The model under review builds one solid part; all positions refer to its coordinate system, in mm. A direction names the side the tool comes from. Round coordinates to 2 decimals unless told otherwise and drop trailing zeros. Order: outer loops, then holes, each group sorted by start corner. A loop starts at its lowest first (then second) coordinate and runs counter-clockwise, first axis right, second up.
from build123d import *

# Parameters (mm, degrees)
SKETCH_1_W      = 23
SKETCH_1_H      = 12.5
EXTRUDE_1_DEPTH = 20
SKETCH_2_W      = 32
SKETCH_2_H      = 12.5
SKETCH_2_R      = 1
EXTRUDE_2_DEPTH = 3
SKETCH_4_R      = 6.25
EXTRUDE_3_DEPTH = 6
SKETCH_5_R      = 2
EXTRUDE_4_DEPTH = 4


with BuildPart() as part:
    # 草图1 → 凸台-拉伸1 (new body)
    with BuildSketch(Plane(origin=(0, 0, 0), x_dir=(1, 0, 0), z_dir=(0, 1, 0))):
        Rectangle(SKETCH_1_W, SKETCH_1_H)
    extrude(amount=EXTRUDE_1_DEPTH)

    # 草图2 → 凸台-拉伸2 (add)
    with BuildSketch(Plane(origin=(0, 20, 0), x_dir=(1, 0, 0), z_dir=(0, 1, 0))):
        Rectangle(SKETCH_2_W, SKETCH_2_H)
        with Locations(Location((13.85, 0, 0), (0, 0, 270))):
            Circle(SKETCH_2_R, mode=Mode.SUBTRACT)
        with Locations(Location((-13.85, 0, 0), (0, 0, 90))):
            Circle(SKETCH_2_R, mode=Mode.SUBTRACT)
    extrude(amount=EXTRUDE_2_DEPTH)

    # 草图4 → 凸台-拉伸3 (add)
    with BuildSketch(Plane(origin=(0, 23, 0), x_dir=(1, 0, 0), z_dir=(0, 1, 0))):
        with Locations(Location((5.25, 0, 0), (0, 0, 270))):
            Circle(SKETCH_4_R)
    extrude(amount=EXTRUDE_3_DEPTH)

    # 草图5 → 凸台-拉伸4 (add)
    with BuildSketch(Plane(origin=(0, 29, 0), x_dir=(1, 0, 0), z_dir=(0, 1, 0))):
        with Locations(Location((5.25, 0, 0), (0, 0, 270))):
            Circle(SKETCH_5_R)
    extrude(amount=EXTRUDE_4_DEPTH)


solid = part.part
(1) We need section B-B (z = 0). Give the boundary of the cut face in (x, y), and give its area (3 significant figures).
(2) Tool access review of faces 5 (the flat face through (3, 29, 0)), 6 (the flat face through (-11.5, 10, 0)), 7 (the flat face through (12.7, 20, -0.1)), 8 (the flat face through (-16, 21, 0)): name each direction out of +Z, -Z, +X, -X, +Y, -Y from which nothing blocks a thin tool from reaching the whole face with its end or side.
(3) We need section C-C (x = 1.5). Give the boundary of the cut face in (y, z), and give its area (4 significant figures).
(4) We need section D-D (y = 22.5). Give the boundary of the cut face in (x, z), and give its area (3 significant figures).
(5) Clearance check with flat-ended pins moving along their axes: P1, Ø2, axis at y = 6, z = 4.5, coming from the +X side; P2, Ø4, axis at x = -3, z = 1, coming from the +Y side; P3, Ø3.5, axis at x = -14, z = -0.5, coming from the -Y side. State where each tip first meets the part, or that it passes through.
(6) To check wall thickness, follow L1, parallel to X at y = 21.5, z = 0; L2, parallel to Z at x = -13.85, y = 22.2; L3, parallel to X at y = 12, z = -4.75. State the ranges of each line that lie inside material, in increasing order.
(7) We need section A-A (x = 13.85). Give the boundary of the cut face in (y, z), and give its area (3 significant figures).
(8) The part is to be moulded in two halves that separate along Z. For faces 1 (the cylindrical face through (12.874, 21.479, -0.217)), 2 (the cylindrical face through (7.233, 30.972, -0.26)), 3 (the flat face through (11.5, 10, 0)), 4 (the cylindrical face through (-12.874, 21.479, 0.217)), say which applies: pulls with the +Z half, pulls with the -Z half, needs draft (parallel to the pull), parting line crosses it, or undercut.
Verdict:
1. outline: (-16, 20) - (-14.85, 20) - (-14.85, 23) - (-16, 23) - close; (-12.85, 20) - (-11.5, 20) - (-11.5, 0) - (11.5, 0) - (11.5, 20) - (12.85, 20) - (12.85, 23) - (11.5, 23) - (11.5, 29) - (7.25, 29) - (7.25, 33) - (3.25, 33) - (3.25, 29) - (-1, 29) - (-1, 23) - (-12.85, 23) - close; (14.85, 20) - (16, 20) - (16, 23) - (14.85, 23) - close
1. area: 635 mm2
2. face 5: +Y
2. face 6: +Z, -Z, -X, -Y
2. face 7: +Z, -Z, +X, -Y
2. face 8: +Z, -Z, -X, +Y, -Y
3. outline: (0, -6.25) - (23, -6.25) - (23, -5) - (29, -5) - (29, 5) - (23, 5) - (23, 6.25) - (0, 6.25) - close
3. area: 347.5 mm2
4. outline: (-16, -6.25) - (16, -6.25) - (16, 6.25) - (-16, 6.25) - close; hole circle Ø2 at (-13.85, 0); hole circle Ø2 at (13.85, 0)
4. area: 394 mm2
5. P1: stops at x = 11.5
5. P2: stops at y = 23
5. P3: stops at y = 20
6. L1: x = -16 to -14.85, -12.85 to 12.85, 14.85 to 16
6. L2: z = -6.25 to -1, 1 to 6.25
6. L3: x = -11.5 to 11.5
7. outline: (20, -6.25) - (23, -6.25) - (23, -1) - (20, -1) - close; (20, 1) - (23, 1) - (23, 6.25) - (20, 6.25) - close
7. area: 31.5 mm2
8. face 1: undercut
8. face 2: parting line crosses it
8. face 3: needs draft
8. face 4: undercut
